```python
from build123d import *

# Parameters (mm, degrees)
F0_W     = 228.6
F0_H     = 228.6
F0_R     = 3
F0_R_2   = 5.08
F1_DEPTH = 10
F2_R     = 25.4


with BuildPart() as f1:
    # F0 (on Front) → F1 (new body)
    with BuildSketch(Plane.XZ):
        Rectangle(F0_W, F0_H)
        with Locations((-90.537816, -86.794242)):
            Circle(F0_R, mode=Mode.SUBTRACT)
        with Locations((-56.537816, -86.794242)):
            Circle(F0_R, mode=Mode.SUBTRACT)
        with Locations((-90.537816, -52.794242)):
            Circle(F0_R, mode=Mode.SUBTRACT)
        with Locations((-56.537816, -52.794242)):
            Circle(F0_R, mode=Mode.SUBTRACT)
        with BuildLine():
            ThreePointArc((-7.422443, 7.396804), (-18.143127, 13.760824), (-24.544206, 24.459424))
            ThreePointArc((-24.544206, 24.459424), (-3.899198, 56.883584), (25.186284, 31.752383))
            ThreePointArc((25.186284, 31.752383), (14.985928, 11.402179), (-7.422443, 7.396804))
        make_face(mode=Mode.SUBTRACT)
        with BuildLine():
            ThreePointArc((-72.865814, 72.614118), (-81.159114, 78.139971), (-71.384126, 76.2))
            ThreePointArc((-71.384126, 76.2), (-71.769138, 74.260029), (-72.865814, 72.614118))
        make_face(mode=Mode.SUBTRACT)
        with Locations((-28.156495, 104.09138)):
            Circle(F0_R_2, mode=Mode.SUBTRACT)
        with Locations((27.624831, 104.092209)):
            Circle(F0_R_2, mode=Mode.SUBTRACT)
        with Locations((75.93329, 76.202263)):
            Circle(F0_R_2, mode=Mode.SUBTRACT)
    extrude(amount=F1_DEPTH)

    # F2
    f2_edges = [f1.edges().sort_by_distance(p)[0] for p in [
        (114.3, -5, 114.3),
        (-114.3, -5, 114.3),
    ]]
    fillet(f2_edges, radius=F2_R)


solid = f1.part
```
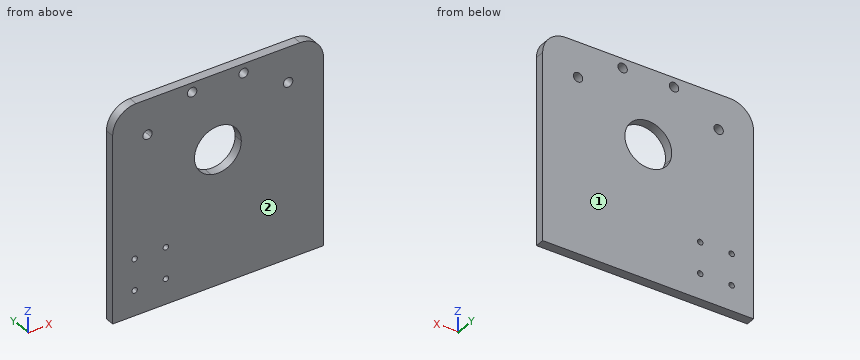
Can you work these out from the model? Positions are in its coordinate system, mm. Face numbers are marked on the shaded views. Coordinates: 2 decimals unless noted, no trailing zeros. Write each question's results on one line, items separated by ' | '.
Item 1: I want a section at A-A, the plane y = -8.25. Count the separate pieces of the cut face and the enclosed holes in it, then the cut area to 3 significant figures.
Results are:
separate pieces: 1 | enclosed holes: 9 | area: 49,500 mm²
Item 2: If I drill on line 1 along X through (y, z) = (-1, 78); line 2 along Z through (x, y) = (5.5, -5.75); line 3 along Z through (x, y) = (71.5, -8), over which ranges is the centre line in solid material (lowest first)?
Results are:
line 1: -114.3 to -81.21, -71.71 to 71.18, 80.68 to 114.3 | line 2: -114.3 to 7, 56.5 to 114.3 | line 3: -114.3 to 73.72, 78.68 to 114.3
Item 3: If we mould it in two halves opening along Y, with no side actions, what happens to the marked faces 1 and 2? For each: +Y half, -Y half, draft (parallel to the pull), parting line (faces both ways), or undercut.
Results are:
face 1: +Y half | face 2: -Y half
